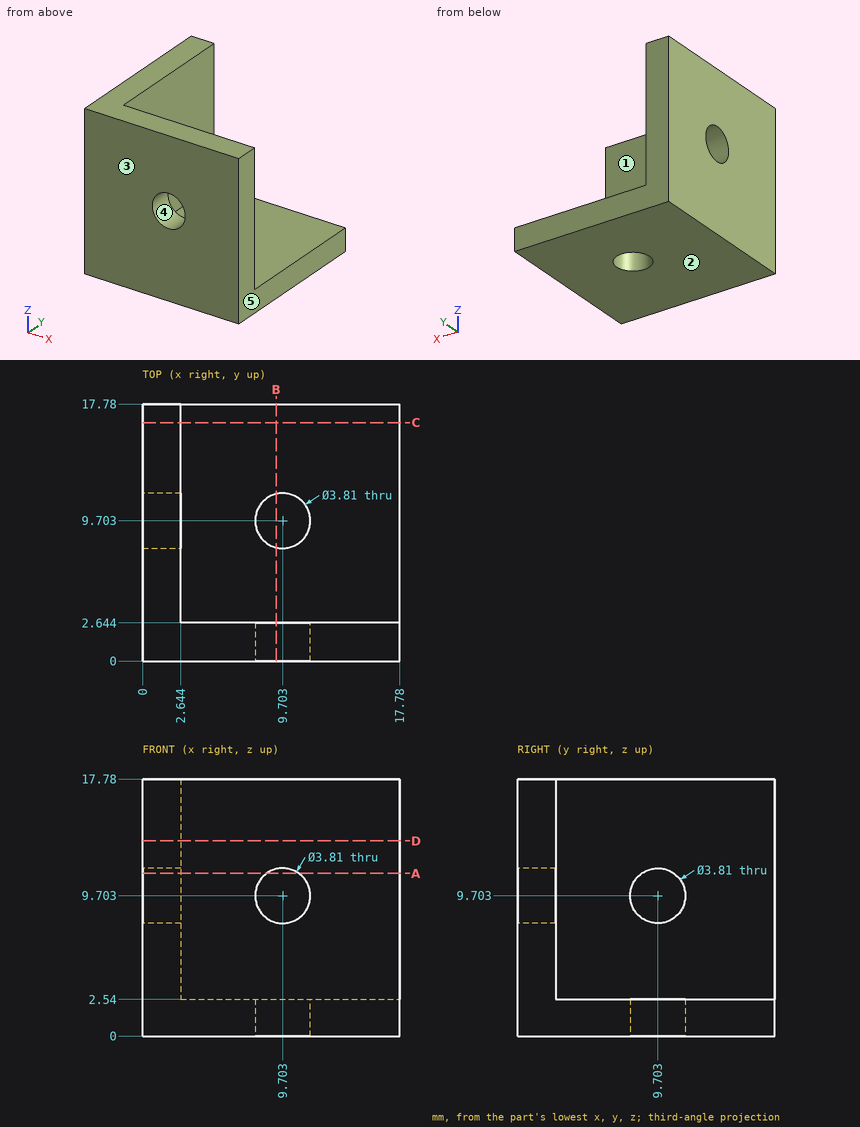
Geometry: see drawing. Coordinates: mm, zero at the bounding-box minimum. A direction names the side the tool comes from. Coordinates: 2 decimals unless noted, no trailing zeros. Write each loop counter-clockwise with the first axis right and the second up, starting at its lowest first coordinate (ties: lowest second). Pieces come first, ordered by that corner, then holes.
1) Section B-B on x = 9.25. Output: boundary loops of the cut face in (y, z).
2) Section C-C on y = 16.5. Output: boundary loops of the cut face in (x, z).
3) Section A-A on z = 11.25. Output: boundary loops of the cut face in (x, y).
4) Section D-D on z = 13.5. Output: boundary loops of the cut face in (x, y).
5) Mould query, pull axis X, two halves, no side actions, for the marked faces 3, 4 and 5. Classes: pulls with the +X half, pulls with the -X half, needs draft (parallel to the pull), parting line crosses it, or undercut.
6) Pin query (flat end, axial travel): pin 1 Ø8 at (x, z) = (15, 2.5) entering from -Y; pin 2 Ø7.5 at (x, y) = (10.5, 7.5) entering from +Z; pin 3 Ø5 at (y, z) = (8.5, 14.5) entering from +X; pin 4 Ø6 at (x, z) = (16, 13.5) entering from +Y. Return the tip coordinate at first contact, or that it passes through.
7) Material intervals for line 1 along X through (y, z) = (16.5, 4); line 2 along Z through (x, y) = (10, 14.75), sorted ascending.
8) Set-up query: the marked faces 1 and 2. Return all of +Z, -Z, +X, -X, +Y, -Y with unobstructed straight access to the full face (end or side cutting, diameter ignored); none if empty.
Check result:
1. outline: (0, 0) - (7.85, 0) - (7.85, 2.54) - (2.64, 2.54) - (2.64, 7.85) - (0, 7.85) - close; (0, 11.55) - (2.64, 11.55) - (2.64, 17.78) - (0, 17.78) - close; (11.55, 0) - (17.78, 0) - (17.78, 2.54) - (11.55, 2.54) - close
2. outline: (0, 0) - (17.78, 0) - (17.78, 2.54) - (2.64, 2.54) - (2.64, 17.78) - (0, 17.78) - close
3. outline: (0, 0) - (8.59, 0) - (8.59, 2.64) - (2.64, 2.64) - (2.64, 8.59) - (0, 8.59) - close; (0, 10.81) - (2.64, 10.81) - (2.64, 17.78) - (0, 17.78) - close; (10.81, 0) - (17.78, 0) - (17.78, 2.64) - (10.81, 2.64) - close
4. outline: (0, 0) - (17.78, 0) - (17.78, 2.64) - (2.64, 2.64) - (2.64, 17.78) - (0, 17.78) - close
5. face 3: needs draft
5. face 4: undercut
5. face 5: pulls with the +X half
6. pin 1: stops at y = 0
6. pin 2: stops at z = 2.54
6. pin 3: stops at x = 2.64
6. pin 4: stops at y = 2.64
7. line 1: x = 0 to 2.64
7. line 2: z = 0 to 2.54
8. face 1: +Z, +X, +Y
8. face 2: -Z, +X, -X, +Y, -Y
